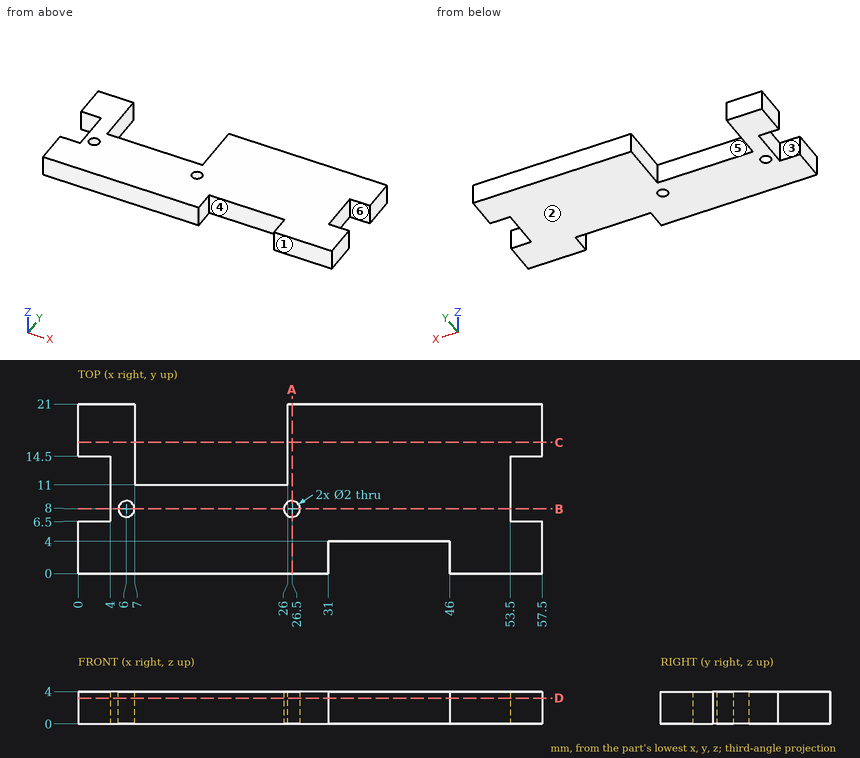
Answer from the drawing. Dimensions are ordinates in mm from the lowest x, y and z of the part. A direction names the side the tool comes from. Round coordinates to 2 decimals unless told otherwise and drop trailing zeros. Write each loop counter-clockwise with the first axis right and the second up, starting at its lowest first coordinate (ties: lowest second). Pieces come first, ordered by that corner, then holes. Notation, with made-up numbers: M 40.25,16.5 L 48.25,16.5 A17 cw 48.25,42.5 Z; hole C 16,-24.5 d6. An arc over 180 degrees is marked long. Write each question's results on one line, items separated by ' | '. Start each with the question number.
Item 1: Find section D-D on z = 3.2. Write down the section's boundary in (x, y), and give its area (3 significant figures).
Item 2: Which of the six approach directions +Z, -Z, +X, -X, +Y, -Y give full straight-line access (tool end or side, diameter ignored) to the marked faces 4, 5 and 6?
Item 3: The mould has two halves that part along Y. Classify the marked faces 1, 2 and 3: +Y half, -Y half, draft (parallel to the pull), parting line (faces both ways), or undercut.
Item 4: Find section C-C on y = 16.25. Write down the section's boundary in (x, z), and give its area (3 significant figures).
Item 5: Find section A-A on x = 26.5. Write down the section's boundary in (y, z).
Item 6: Find section B-B on y = 8. Write down the section's boundary in (x, z), and give its area (3 significant figures).
Item 7: Straight lines are drawn through the part: probe 1 along X at (y, z) = (11.25, 1.25); probe 2 along Y at (x, z) = (26.5, 1.4); probe 3 along X at (y, z) = (15.25, 0.6). For each, find the intervals that lie inside material, in ascending order.
Item 8: Given pin 1 Ø2.5 at (x, y) = (26.5, 8) entering from +Z; pin 2 Ø1.2 at (x, z) = (37.5, 1.5) entering from -Y; pin 3 Ø2 at (x, z) = (18.5, 2) entering from +Y; pin 4 Ø2 at (y, z) = (8.5, 2.5) entering from -X, each flat-ended and moving along its own axis, determine where each tip first touches the part or whether it passes through.
Answer block:
1) outline: M 0,0 L 31,0 L 31,4 L 46,4 L 46,0 L 57.5,0 L 57.5,6.5 L 53.5,6.5 L 53.5,14.5 L 57.5,14.5 L 57.5,21 L 26,21 L 26,11 L 7,11 L 7,21 L 0,21 L 0,14.5 L 4,14.5 L 4,6.5 L 0,6.5 Z; hole C 6,8 d2; hole C 26.5,8 d2 | area: 887 mm²
2) face 4: +Z, -Z, -Y | face 5: +Z, -Z, +Y | face 6: +Z, -Z, +X
3) face 1: -Y half | face 2: draft | face 3: undercut
4) outline: M 0,0 L 7,0 L 7,4 L 0,4 Z; M 26,0 L 57.5,0 L 57.5,4 L 26,4 Z | area: 154 mm²
5) outline: M 0,0 L 7,0 L 7,4 L 0,4 Z; M 9,0 L 21,0 L 21,4 L 9,4 Z
6) outline: M 4,0 L 5,0 L 5,4 L 4,4 Z; M 7,0 L 25.5,0 L 25.5,4 L 7,4 Z; M 27.5,0 L 53.5,0 L 53.5,4 L 27.5,4 Z | area: 182 mm²
7) probe 1: x = 4 to 7, 26 to 53.5 | probe 2: y = 0 to 7, 9 to 21 | probe 3: x = 0 to 7, 26 to 57.5
8) pin 1: stops at z = 4 | pin 2: stops at y = 4 | pin 3: stops at y = 11 | pin 4: stops at x = 4
